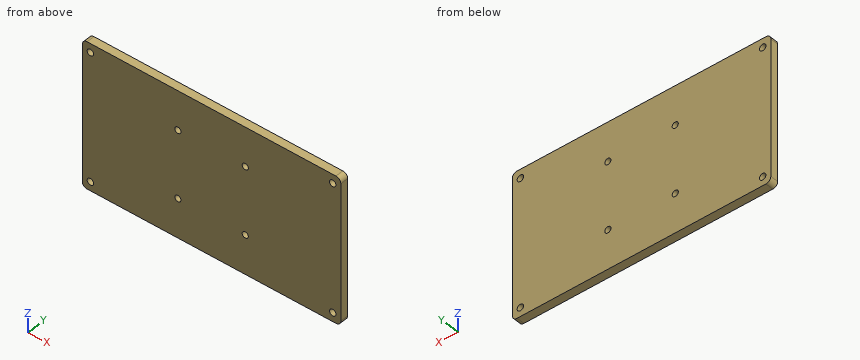
```python
from build123d import *

# Parameters (mm, degrees)
SKETCH_1_W      = 160
SKETCH_1_H      = 90
SKETCH_1_R      = 1.9
SKETCH_1_R_2    = 2
EXTRUDE_1_DEPTH = 5
FILLET_5_R      = 3


with BuildPart() as part:
    # Эскиз1 → Бобышка-Вытянуть1 (new body)
    with BuildSketch(Plane(origin=(0, 0, 0), x_dir=(1, 0, 0), z_dir=(0, 1, 0))):
        Rectangle(SKETCH_1_W, SKETCH_1_H)
        with Locations(Location((20.859650045, 20.859650045, 0), (0, 0, 270))):
            Circle(SKETCH_1_R, mode=Mode.SUBTRACT)
        with Locations(Location((20.859650045, -20.859650045, 0), (0, 0, 270))):
            Circle(SKETCH_1_R, mode=Mode.SUBTRACT)
        with Locations(Location((-20.859650045, -20.859650045, 0), (0, 0, 270))):
            Circle(SKETCH_1_R, mode=Mode.SUBTRACT)
        with Locations(Location((-20.859650045, 20.859650045, 0), (0, 0, 270))):
            Circle(SKETCH_1_R, mode=Mode.SUBTRACT)
        with Locations(Location((-75, 39.5, 0), (0, 0, 270))):
            Circle(SKETCH_1_R_2, mode=Mode.SUBTRACT)
        with Locations(Location((75, 39.5, 0), (0, 0, 270))):
            Circle(SKETCH_1_R_2, mode=Mode.SUBTRACT)
        with Locations(Location((75, -39.5, 0), (0, 0, 270))):
            Circle(SKETCH_1_R_2, mode=Mode.SUBTRACT)
        with Locations(Location((-75, -39.5, 0), (0, 0, 270))):
            Circle(SKETCH_1_R_2, mode=Mode.SUBTRACT)
    extrude(amount=EXTRUDE_1_DEPTH)

    # Скругление5
    fillet_5_edges = [part.edges().sort_by_distance(p)[0] for p in [
        (80, 2.5, 45),
        (-80, 2.5, 45),
        (-80, 2.5, -45),
        (80, 2.5, -45),
    ]]
    fillet(fillet_5_edges, radius=FILLET_5_R)


solid = part.part
```
For this review, take the finished solid that the model builds, in its own axes (mm). Round coordinates to 2 decimals unless told otherwise and drop trailing zeros. Loops run counter-clockwise (first coordinate to the right, second up) from the corner with the lowest first, then second, coordinate; pieces in that order, holes last.
(1) We need section A-A (z = 39.5). Give the boundary of the cut face in (x, y), plus the area to 3 significant figures.
Returned:
outline: (-80, 0) - (-77, 0) - (-77, 5) - (-80, 5) - close; (-73, 0) - (73, 0) - (73, 5) - (-73, 5) - close; (77, 0) - (80, 0) - (80, 5) - (77, 5) - close
area: 760 mm2
(2) We need section B-B (x = 75). Give the boundary of the cut face in (y, z), plus the area to 3 significant figures.
Returned:
outline: (0, -45) - (5, -45) - (5, -41.5) - (0, -41.5) - close; (0, -37.5) - (5, -37.5) - (5, 37.5) - (0, 37.5) - close; (0, 41.5) - (5, 41.5) - (5, 45) - (0, 45) - close
area: 410 mm2
(3) Clearance check with a flat-ended pin moving along its axis: P1, Ø1.5, axis at x = 35.5, z = -6, coming from the -Y side. State where the tip first meets the part, or that it passes through.
Returned:
P1: stops at y = 0
(4) Wall thickness on line 1 along X through (y, z) = (2.15, 39.5); line 2 along Z through (x, y) = (-20, 4.7); line 3 along X through (y, z) = (0.25, 22.5): over which ranges is each line inside the solid? List them lowest first.
Returned:
line 1: x = -80 to -77, -73 to 73, 77 to 80
line 2: z = -45 to -22.55, -19.17 to 19.17, 22.55 to 45
line 3: x = -80 to -21.82, -19.9 to 19.9, 21.82 to 80
